from build123d import *

# Parameters (mm, degrees)
F0_W     = 10.16
F0_H     = 76.2
F1_DEPTH = 31.75
F3_D     = 17.78
F3_DEPTH = 12.7
F5_D     = 17.78
F5_DEPTH = 12.7


with BuildPart() as f1:
    # F0 (on Front) → F1 (new body, symmetric)
    with BuildSketch(Plane.XZ):
        with Locations((-81.28, 43.18)):
            Rectangle(F0_W, F0_H)
        with Locations((81.28, 43.18)):
            Rectangle(F0_W, F0_H)
        Polygon((-76.2, 5.08), (-86.36, 5.08), (-86.36, -5.08), (86.36, -5.08), (86.36, 5.08), (76.2, 5.08), align=None)
    extrude(amount=F1_DEPTH, both=True)

    # F3
    with Locations(Plane.YZ.offset(86.36)):
        with Locations((11.43, 35.56)):
            Hole(F3_D / 2, depth=F3_DEPTH)

    # F5
    with Locations(Plane(origin=(-86.36, 0, 0), x_dir=(0, -1, 0), z_dir=(-1, 0, 0))):
        with Locations((11.43, 60.96)):
            Hole(F5_D / 2, depth=F5_DEPTH)


solid = f1.part
Geometry check sheet. Reference: the model listing, model coordinates, mm. A direction names the side the tool comes from. Give positions to 0.01 mm unless a question says otherwise; leave off trailing zeros. Order: outer loops, then holes, each group sorted by start corner. A loop starts at its lowest first (then second) coordinate and runs counter-clockwise, first axis right, second up. Notation, with made-up numbers: (-15, 23) - (1, 23) arc R13 cw to (1, 48) - close; hole circle Ø5 at (49, -2.75). An arc over 180 degrees is marked (long way). Answer as a JSON object with one key per item and string values.
(1) Draft check along Z on faces 1 (the flat face through (-81, 0, 81.28)), 2 (the flat face through (86.36, 0, 37)), 3 (the cylindrical face through (-81.21, -13.36, 52.28)). Enter one of: released by +Z, released by -Z, zero draft, split by the parting line, or undercut.
Report:
{"face 1": "released by +Z", "face 2": "zero draft", "face 3": "undercut"}
(2) Material ranges on line 1 (X direction, y = 17, z = 59.5); line 2 (Z direction, x = 79, y = 11); line 3 (Z direction, x = -83, y = -11), recorded low to high.
Report:
{"line 1": "-86.36 to -76.2, 76.2 to 86.36", "line 2": "-5.08 to 26.68, 44.44 to 81.28", "line 3": "-5.08 to 52.08, 69.84 to 81.28"}
(3) Cross-section at D-D (y = -25.5). Record the cut outline in (x, z), then the cut area to 3 significant figures.
Report:
{"outline": "(-86.36, -5.08) - (86.36, -5.08) - (86.36, 81.28) - (76.2, 81.28) - (76.2, 5.08) - (-76.2, 5.08) - (-76.2, 81.28) - (-86.36, 81.28) - close", "area": "3,300 mm^2"}
(4) Cross-section at B-B (y = 11.43). Record the cut outline in (x, z), then the cut area to 3 significant figures.
Report:
{"outline": "(-86.36, -5.08) - (86.36, -5.08) - (86.36, 26.67) - (76.2, 26.67) - (76.2, 5.08) - (-76.2, 5.08) - (-76.2, 81.28) - (-86.36, 81.28) - close; (76.2, 44.45) - (86.36, 44.45) - (86.36, 81.28) - (76.2, 81.28) - close", "area": "3,120 mm^2"}
(5) Cross-section at A-A (z = 18). Record the cut outline in (x, y).
Report:
{"outline": "(-86.36, -31.75) - (-76.2, -31.75) - (-76.2, 31.75) - (-86.36, 31.75) - close; (76.2, -31.75) - (86.36, -31.75) - (86.36, 31.75) - (76.2, 31.75) - close"}
(6) Tool access check on faces 4 (the flat face through (1, 0, 5.08)), 5 (the flat face through (6, -31.75, 3)), 6 (the cylindrical face through (81.209, 12.587, 44.374)). Record the directions out of +Z, -Z, +X, -X, +Y, -Y that give a thin tool (end or side, any length) a straight path to the whole face; none if there is none.
Report:
{"face 4": "+Z, +Y, -Y", "face 5": "+Z, -Z, +X, -X, -Y", "face 6": "+X"}
(7) Cross-section at C-C (z = 60.96). Record the cut outline in (x, y), then the cut area to 3 significant figures.
Report:
{"outline": "(-86.36, -31.75) - (-76.2, -31.75) - (-76.2, -20.32) - (-86.36, -20.32) - close; (-86.36, -2.54) - (-76.2, -2.54) - (-76.2, 31.75) - (-86.36, 31.75) - close; (76.2, -31.75) - (86.36, -31.75) - (86.36, 31.75) - (76.2, 31.75) - close", "area": "1,110 mm^2"}
(8) Depth check by flat-ended pin: pin 1 Ø20.5 at (y, z) = (-11.43, 60.96) entering from -X; pin 2 Ø19 at (x, y) = (-10.5, 10.5) entering from +Z; pin 3 Ø3 at (y, z) = (-11.5, 60.5) entering from -X. Enter the tip coordinate at first touch or a pass-through.
Report:
{"pin 1": "x = -86.36", "pin 2": "z = 5.08", "pin 3": "x = 76.2"}
